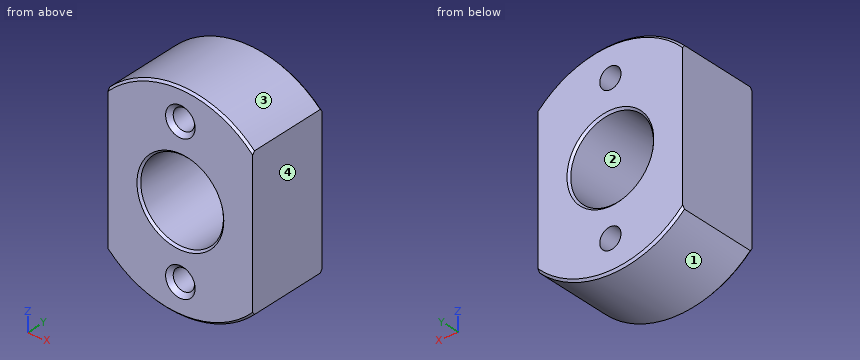
Autodesk Fusion 360 part; units mm, degrees
sketch "Sketch1" plane through (0, 0, 0) normal (0, 1, 0) x (1, 0, 0)
  circle A0 centre (0, 0) radius 20
  line L0 (-35, 35.7071) -> (-35, -35.7071)
  line L1 (0, 0) -> (0, 70.7339) construction
  line L2 (35, 35.7071) -> (35, -35.7071)
  arc A1 (-35, -35.7071) -> (35, -35.7071) centre (0, 0) ccw
  arc A2 (35, 35.7071) -> (-35, 35.7071) centre (0, 0) ccw
  dimension "d1" = 40
  dimension "d2" = 100
  dimension "d3" = 70
  dimension "d6" = 35
extrude "Extrude1" add sketch "Sketch1" along normal mid plane 40
sketch "Sketch2" plane through (0, 20, 0) normal (0, 1, 0) x (-1, 0, 0)
  circle A0 centre (0, 0) radius 20
  arc A1 (-35, -35.7071) -> (35, -35.7071) centre (0, 0) ccw
  line L0 (35, -35.7071) -> (35, 35.7071)
  arc A2 (35, 35.7071) -> (-35, 35.7071) centre (0, 0) ccw
  line L1 (-35, 35.7071) -> (-35, -35.7071)
  circle A3 centre (0, -35) radius 5
  line L2 (0, 0) -> (45, 0) construction
  circle A4 centre (0, 35) radius 5
  dimension "d7" = 10
  dimension "d8" = 35
extrude "Extrude2" cut sketch "Sketch2" against normal blind 80 contours A3 | A4
chamfer "Chamfer1" distance 1 angle 45 3 edges at (0, 20, -50) (0, 20, 50) (-18.6465, 20, -7.2323)
chamfer "Chamfer1" distance 1 angle 45 3 edges at (0, -20, -50) (0, -20, 50) (-18.6465, -20, 7.2323)
hole "Hole1" at (0, -20, -35) direction (0, 1, 0) diameter 10.274 end through all
hole "Hole2" at (0, -20, 35) direction (0, 1, 0) diameter 10.274 end through all
chamfer "Chamfer2" distance 2 angle 45 2 edges at (1.8575, -20, -30.2109) (1.8575, -20, 39.7891)
Could you check a few things on this model? Use its own coordinates, in mm. Face numbers are marked on the shaded views. Give positions to 0.01 mm unless a question says otherwise; leave off trailing zeros. Write each loop counter-clockwise with the first axis right and the second up, starting at its lowest first coordinate (ties: lowest second). Pieces come first, ordered by that corner, then holes. Notation, with made-up numbers: (-33.5, -25.5) -> (23.5, -25.5) arc R23 ccw to (23.5, -4.5) -> close; hole circle Ø5 at (40.25, 57). An arc over 180 degrees is marked (long way). Write each question's results on one line, items separated by ' | '. Start each with the question number.
Q1. Suppose I cut it at C-C, the plane y = -4. List the corners of the cut face in (x, z) for me.
Q2. Suppose I cut it at A-A, the plane z = 0. List the corners of the cut face in (x, y) for me, and give its area (3 significant figures).
Q3. We'd pull the mould along Z, two halves only. Please class the marked faces 1, 2, 3 and 4: +Z half, -Z half, draft (parallel to the pull), parting line (faces both ways), or undercut.
Q4. I'm going to push flat-ended pins straight in: pin 1 Ø13.5 at (x, z) = (0, -35) entering from -Y; pin 2 Ø1.5 at (x, y) = (19, -5) entering from +Z; pin 3 Ø8 at (x, y) = (-15, -3.5) entering from +Z. Where does each tip first touch, or does it pass through?
Q5. I need wall thicknesses on probe 1 along X at (y, z) = (2, 35); probe 2 along X at (y, z) = (-3, 0); probe 3 along Z at (x, y) = (-12, -15). Which ranges of each line are inside material? Lowest first, please.
Q6. Suppose I cut it at B-B, the plane x = 0. List the corners of the cut face in (y, z) for me, and give its area (3 significant figures).
Outcome:
1) outline: (-35, -35.71) arc R50 ccw to (35, -35.71) -> (35, 35.71) arc R50 ccw to (-35, 35.71) -> close; hole circle Ø40 at (0, 0); hole circle Ø10.27 at (0, -35); hole circle Ø10.27 at (0, 35)
2) outline: (-35, -20) -> (-21, -20) -> (-20, -19) -> (-20, 19) -> (-21, 20) -> (-35, 20) -> close; (20, -19) -> (21, -20) -> (35, -20) -> (35, 20) -> (21, 20) -> (20, 19) -> close | area: 1,200 mm2
3) face 1: -Z half | face 2: undercut | face 3: +Z half | face 4: draft
4) pin 1: y = -19.61 | pin 2: z = 46.55 | pin 3: z = 48.77
5) probe 1: -35 to -5.14, 5.14 to 35 | probe 2: -35 to -20, 20 to 35 | probe 3: -48.54 to -16, 16 to 48.54
6) outline: (-20, -49) -> (-19, -50) -> (19, -50) -> (20, -49) -> (20, -40.14) -> (-18, -40.14) -> (-20, -42.14) -> close; (-20, -27.86) -> (-18, -29.86) -> (20, -29.86) -> (20, -21) -> (19, -20) -> (-19, -20) -> (-20, -21) -> close; (-20, 21) -> (-19, 20) -> (19, 20) -> (20, 21) -> (20, 29.86) -> (-18, 29.86) -> (-20, 27.86) -> close; (-20, 42.14) -> (-18, 40.14) -> (20, 40.14) -> (20, 49) -> (19, 50) -> (-19, 50) -> (-20, 49) -> close | area: 1,570 mm2
